Design review of the part built by this model. Coordinates are the model's own, in mm. Face numbers are marked on the shaded views. A direction names the side the tool comes from. Give positions to 0.01 mm unless a question says otherwise; leave off trailing zeros. Loops run counter-clockwise (first coordinate to the right, second up) from the corner with the lowest first, then second, coordinate; pieces in that order, holes last. Notation, with made-up numbers: (20, 65.25) -> (29, 65.25) arc R11 ccw to (29, 81.25) -> close; hole circle Ø4 at (85, 76.25). An arc over 180 degrees is marked (long way). Use a Markdown table: item, result. Add a question column.
1. For the marked faces 4 and 5, list the 3-axis set-ups (+Z, -Z, +X, -X, +Y, -Y) from which the entire face can be reached by the end or side of a thin tool; tool diameter is ignored.
2. Add section A-A (x = 0). State the section outline as (y, z) points.
3. Add section C-C (y = 0). Count the separate pieces of the cut face and the enclosed holes in it, and give its area (3 significant figures).
4. To check wall thickness, follow line 1 (Y direction, x = 0, z = 76); line 2 (Z direction, x = -26, y = 14); line 3 (Y direction, x = -14, z = 1). State the ranges of each line that lie inside material, in increasing order.
5. Draft analysis for pull direction Z (two halves, no side actions). For the marked faces 1, 2 and 3, state which applies: pulls with the +Z half, pulls with the -Z half, needs draft (parallel to the pull), parting line crosses it, or undercut.
6. Add section D-D (x = 22.5). State the section outline as (y, z) points.
7. For pin 1 Ø12.5 at (x, y) = (-2.5, -5) entering from +Z; pin 2 Ø10 at (x, z) = (20, 62.5) entering from -Y; pin 3 Ø10 at (y, z) = (25, 43) entering from -X, all flat-tipped, find the tip position at first contact; note any pin that passes through.
8. Add section B-B (y = 17.5). State the section outline as (x, z) points, and give its area (3 significant figures).
Autodesk Inventor part; units mm, degrees
ref_plane "Work Plane2" through (-15.0271, -15.0271, 76.5) normal (0, 0, -1) x (0, 1, 0)
ref_plane "YZ Plane" through (0, 0, 0) normal (1, 0, 0) x (0, 1, 0)
ref_plane "XZ Plane" through (0, 0, 0) normal (0, 1, 0) x (-1, 0, 0)
ref_plane "Work Plane1" through (0, 0, 0) normal (0, 0, 1) x (1, 0, 0)
sketch "Sketch1" plane through (0, 0, 0) normal (0, 0, 1) x (1, 0, 0)
  line L0 (-37.5, -37.5) -> (37.5, -37.5)
  line L1 (37.5, -37.5) -> (37.5, 37.5)
  line L2 (37.5, 37.5) -> (-37.5, 37.5)
  line L3 (-37.5, 37.5) -> (-37.5, -37.5)
  line L4 (-37.5, -37.5) -> (37.5, 37.5) construction
  line L5 (37.5, -37.5) -> (-37.5, 37.5) construction
  circle A0 centre (14.5, 25.1147) radius 5
  circle A1 centre (-14.5, 25.1147) radius 5
  circle A2 centre (-29, 0) radius 5
  circle A3 centre (29, 0) radius 5
  circle A4 centre (14.5, -25.1147) radius 5
  circle A5 centre (-14.5, -25.1147) radius 5
  point P0 (0, 0)
  dimension "d0" = 75
extrude "Extrusion1" add sketch "Sketch1" along normal blind 2
sketch "Sketch2" plane through (0, 0, 2) normal (0, 0, 1) x (1, 0, 0)
  circle A0 centre (0, 0) radius 40 construction
  line L0 (28.2843, -28.2843) -> (-28.2843, -28.2843) construction
  line L1 (-28.2843, -28.2843) -> (-28.2843, 28.2843) construction
  line L2 (-28.2843, 28.2843) -> (28.2843, 28.2843) construction
  line L3 (28.2843, 28.2843) -> (28.2843, -28.2843) construction
  line L4 (28.2843, -28.2843) -> (-28.2843, 28.2843) construction
  line L5 (-28.2843, -28.2843) -> (28.2843, 28.2843) construction
  circle A1 centre (-28.2843, 28.2843) radius 4
  circle A2 centre (-28.2843, -28.2843) radius 4
  circle A3 centre (28.2843, -28.2843) radius 4
  circle A4 centre (28.2843, 28.2843) radius 4
  dimension "d3" = 80
  dimension "d4" = 8
  dimension "d7" = 360
ref_plane "Work Plane2" through (-15.0271, -15.0271, 76.5) normal (0, 0, -1) x (0, 1, 0)
extrude "Extrusion2" add sketch "Sketch2" along normal up to surface (74.5 mm away)
sketch "Sketch3" plane through (28.2843, 28.2843, 76.5) normal (0, 0, 1) x (1, 0, 0)
  circle A0 centre (-45.7843, -28.2843) radius 2
  circle A1 centre (-28.2843, -10.7843) radius 2
  circle A2 centre (-28.2843, -45.7843) radius 2
  circle A3 centre (-10.7843, -28.2843) radius 2
  circle A4 centre (-28.2843, -28.2843) radius 4
  line L0 (-65.7843, 9.2157) -> (-65.7843, -65.7843)
  line L1 (9.2157, 9.2157) -> (-65.7843, 9.2157)
  line L2 (9.2157, -65.7843) -> (9.2157, 9.2157)
  line L3 (-65.7843, -65.7843) -> (9.2157, -65.7843)
  point P0 (-28.2843, -28.2843)
extrude "Extrusion3" add sketch "Sketch3" against normal blind 1
sketch "Sketch4" plane through (-37.5, -37.5, 76.5) normal (0, 0, 1) x (1, 0, 0)
  line L0 (0, 75) -> (0, 0)
  line L1 (0, 0) -> (75, 0)
  line L2 (75, 0) -> (75, 75)
  line L3 (75, 75) -> (0, 75)
  circle A0 centre (20, 37.5) radius 2
  circle A1 centre (37.5, 55) radius 2
  circle A2 centre (37.5, 20) radius 2
  circle A3 centre (55, 37.5) radius 2
  circle A4 centre (37.5, 37.5) radius 4
  circle A5 centre (37.5, 37.5) radius 12.5
  point P0 (37.5, 37.5)
extrude "Extrusion4" add sketch "Sketch4" along normal blind 1 contours L3 L2 L1 L0
properties part number "mega troque motor to nmrv-50 flange"
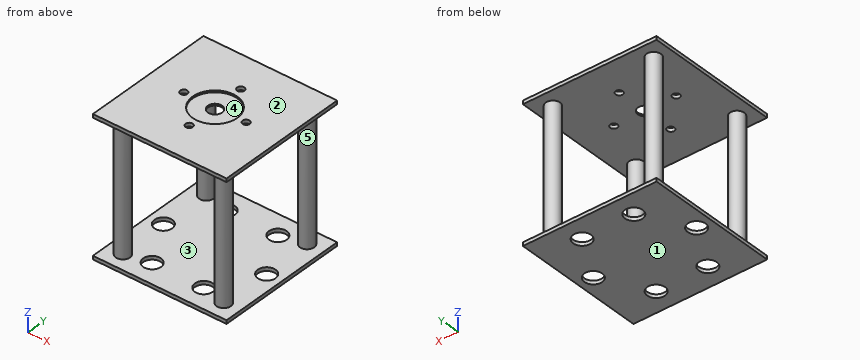
Taken from the geometry:
| question | item | result |
|---|---|---|
| 1 | face 4 | +Z |
| 1 | face 5 | none |
| 2 | outline | (-37.5, 0) -> (37.5, 0) -> (37.5, 2) -> (-37.5, 2) -> close; (-37.5, 75.5) -> (-19.5, 75.5) -> (-19.5, 77.5) -> (-37.5, 77.5) -> close; (-15.5, 75.5) -> (-4, 75.5) -> (-4, 76.5) -> (-12.5, 76.5) -> (-12.5, 77.5) -> (-15.5, 77.5) -> close; (4, 75.5) -> (15.5, 75.5) -> (15.5, 77.5) -> (12.5, 77.5) -> (12.5, 76.5) -> (4, 76.5) -> close; (19.5, 75.5) -> (37.5, 75.5) -> (37.5, 77.5) -> (19.5, 77.5) -> close |
| 3 | separate pieces | 7 |
| 3 | enclosed holes | 0 |
| 3 | area | 211 mm^2 |
| 4 | line 1 | y = -37.5 to -19.5, -15.5 to -4, 4 to 15.5, 19.5 to 37.5 |
| 4 | line 2 | z = 0 to 2, 75.5 to 77.5 |
| 4 | line 3 | y = -37.5 to -30.09, -20.14 to 20.14, 30.09 to 37.5 |
| 5 | face 1 | pulls with the -Z half |
| 5 | face 2 | pulls with the +Z half |
| 5 | face 3 | undercut |
| 6 | outline | (-37.5, 0) -> (37.5, 0) -> (37.5, 2) -> (-37.5, 2) -> close; (-37.5, 75.5) -> (37.5, 75.5) -> (37.5, 77.5) -> (-37.5, 77.5) -> close |
| 7 | pin 1 | stops at z = 76.5 |
| 7 | pin 2 | stops at y = -30.57 |
| 7 | pin 3 | stops at x = -32.28 |
| 8 | outline | (-37.5, 0) -> (37.5, 0) -> (37.5, 2) -> (-37.5, 2) -> close; (-37.5, 75.5) -> (-2, 75.5) -> (-2, 77.5) -> (-37.5, 77.5) -> close; (2, 75.5) -> (37.5, 75.5) -> (37.5, 77.5) -> (2, 77.5) -> close |
| 8 | area | 292 mm^2 |
